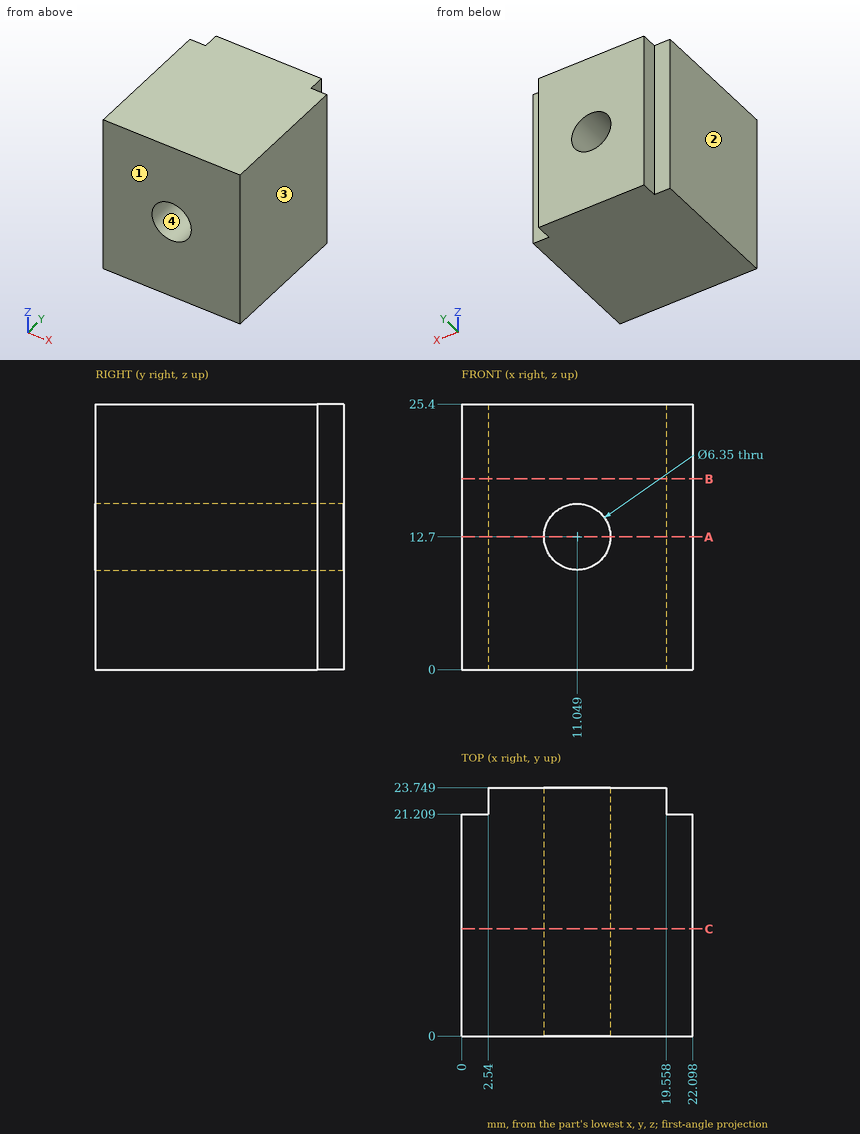
Can you work these out from the drawing? Everything is in mm from the part's minimum corner. Round coordinates to 2 decimals unless told otherwise and drop trailing zeros. Loops run counter-clockwise (first coordinate to the right, second up) from the corner with the lowest first, then second, coordinate; pieces in that order, holes last. Notation, with made-up numbers: (37, 66.25) - (91, 66.25) arc R20 ccw to (91, 92.25) - close; hole circle Ø7 at (22, 37). An arc over 180 degrees is marked (long way). Write item = value, one per line. Start each with the question number.
(1) If we section it at B-B (z = 18.25): Please give me the cut outline in (x, y).
(2) For P1, Ø4, axis at x = 2.5, y = 17.5, coming from the -Z side; P2, Ø0.8, axis at y = 22.5, z = 10.5, coming from the +X side; P3, Ø0.8, axis at x = 21, z = 7, coming from the +Y side, each with a flat end and sliding along its axis, tell me the tip position at first contact or that it passes through.
(3) If we mould it in two halves opening along X, with no side actions, what happens to the marked faces 1, 2, 3 and 4? For each: released by +X, released by -X, zero draft, split by the parting line, or undercut.
(4) If we section it at A-A (z = 12.7): Please give me the cut outline in (x, y).
(5) If we section it at C-C (y = 10.25): Please give me the cut outline in (x, z) (3 decimals).
(6) If I drill on probe 1 along Z at (x, y) = (11.25, 17.25); probe 2 along X at (y, z) = (11, 12.7); probe 3 along Z at (x, y) = (9.5, 18), over which ranges is the centre line in solid material (lowest first)? Write a range as [from, to].
Ans:
q1.outline = (0, 0) - (22.1, 0) - (22.1, 21.21) - (19.56, 21.21) - (19.56, 23.75) - (2.54, 23.75) - (2.54, 21.21) - (0, 21.21) - close
q2.P1 = 0
q2.P2 = 19.56
q2.P3 = 21.21
q3.face_1 = zero draft
q3.face_2 = released by -X
q3.face_3 = released by +X
q3.face_4 = undercut
q4.outline = (0, 0) - (7.87, 0) - (7.87, 23.75) - (2.54, 23.75) - (2.54, 21.21) - (0, 21.21) - close; (14.22, 0) - (22.1, 0) - (22.1, 21.21) - (19.56, 21.21) - (19.56, 23.75) - (14.22, 23.75) - close
q5.outline = (0, 0) - (22.098, 0) - (22.098, 25.4) - (0, 25.4) - close; hole circle Ø6.35 at (11.049, 12.7)
q6.probe_1 = [0, 9.53], [15.87, 25.4]
q6.probe_2 = [0, 7.87], [14.22, 22.1]
q6.probe_3 = [0, 9.93], [15.47, 25.4]
